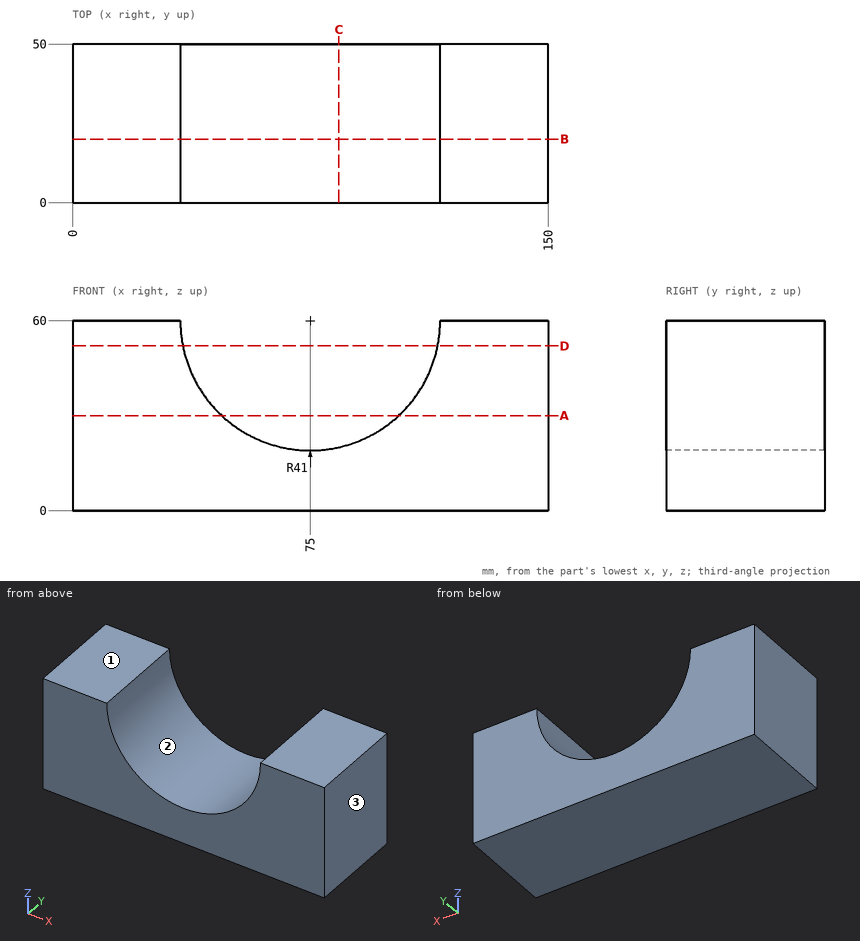
Source: three-view drawing plus pictorial views. Frame: mm from the lowest corner of the part. Give positions to 0.01 mm unless a question says otherwise; leave off trailing zeros. Loops run counter-clockwise (first coordinate to the right, second up) from the corner with the lowest first, then second, coordinate; pieces in that order, holes last. Notation, with made-up numbers: M 5,1.5 L 56,1.5 A24 ccw 56,19.5 Z; hole C 3.5,34 d7. An arc over 180 degrees is marked long. Put each result on its own line as item: value.
Q1. Mould query, pull axis X, two halves, no side actions, for the marked faces 1, 2 and 3. Classes: released by +X, released by -X, zero draft, split by the parting line, or undercut.
Response values:
face 1: zero draft
face 2: undercut
face 3: released by +X
Q2. Line query: probe 1 along X at (y, z) = (14, 49.5); probe 2 along X at (y, z) = (3, 24.5); probe 3 along Z at (x, y) = (76, 4). Output: solid intervals per line, ascending. Write a range as [from, to].
Response values:
probe 1: x = [0, 35.37], [114.63, 150]
probe 2: x = [0, 54.49], [95.51, 150]
probe 3: z = [0, 19.01]
Q3. Section A-A (z = 30). Return the cut outline in (x, y).
Response values:
outline: M 0,0 L 47.05,0 L 47.05,50 L 0,50 Z; M 102.95,0 L 150,0 L 150,50 L 102.95,50 Z
Q4. Section C-C (x = 84). Return the cut outline in (y, z), and give its area (3 significant figures).
Response values:
outline: M 0,0 L 50,0 L 50,20 L 0,20 Z
area: 1,000 mm²
Q5. Section D-D (z = 52). Return the cut outline in (x, y), and give its area (3 significant figures).
Response values:
outline: M 0,0 L 34.79,0 L 34.79,50 L 0,50 Z; M 115.21,0 L 150,0 L 150,50 L 115.21,50 Z
area: 3,480 mm²
Q6. Section B-B (y = 20). Return the cut outline in (x, z), and give its area (3 significant figures).
Response values:
outline: M 0,0 L 150,0 L 150,60 L 116,60 A41 cw 34,60 L 0,60 Z
area: 6,360 mm²
Q7. Pin query (flat end, axial travel): P1, Ø6, axis at x = 72, y = 29, coming from the +Z side. Return the tip coordinate at first contact, or that it passes through.
Response values:
P1: stops at z = 19.44
